Part print with two shaded views. Sizes in mm from the minimum x, y, z corner. A direction names the side the tool comes from. Round coordinates to 2 decimals unless told otherwise and drop trailing zeros. Loops run counter-clockwise (first coordinate to the right, second up) from the corner with the lowest first, then second, coordinate; pieces in that order, holes last. Notation, with made-up numbers: (87, 51.25) -> (107, 51.25) arc R23 ccw to (107, 63.25) -> close; hole circle Ø9 at (-19.75, 73). An arc over 180 degrees is marked (long way). Use a Markdown table: item, result. Add a question column.
Item 1: Cut at A-A, the plane z = 16.5. List the corners of the cut face in (x, y).
Item 2: Cut at B-B, the plane z = 69. List the corners of the cut face in (x, y), plus the area to 3 significant figures.
Item 3: Flat gauge pins, fed straight in: pin 1 (12 mm diameter, centred on y = 49.5, z = 14, fed in from +X); pin 2 (3 mm diameter, centred on x = 17.5, z = 39.5, fed in from +Y) (1 decimal); pin 3 (6 mm diameter, centred on x = 18.5, y = 35, fed in from +Z); pin 4 (8 mm diameter, centred on x = 31, y = 8, fed in from -Z). Where does each tip first touch, or does it go through?
Item 4: Probe line 1 (X direction, y = 15.5, z = 17) (1 decimal); line 2 (Z direction, x = 26, y = 18); line 3 (Y direction, x = 58, z = 15) (1 decimal). List the from-to ranges inside material, lowest first. Write a range as [from, to].
Item 5: Two-plate mould, pull along Y, no slides. Class the marked faces 3, 4, 5 and 6: pulls with the +Y half, pulls with the -Y half, needs draft (parallel to the pull), parting line crosses it, or undercut.
Item 6: Which spindle directions (+Z, -Z, +X, -X, +Y, -Y) get a long thin tool onto all of the face, cutting with end or side? Do the marked faces 1 and 2. Say none if no direction does.
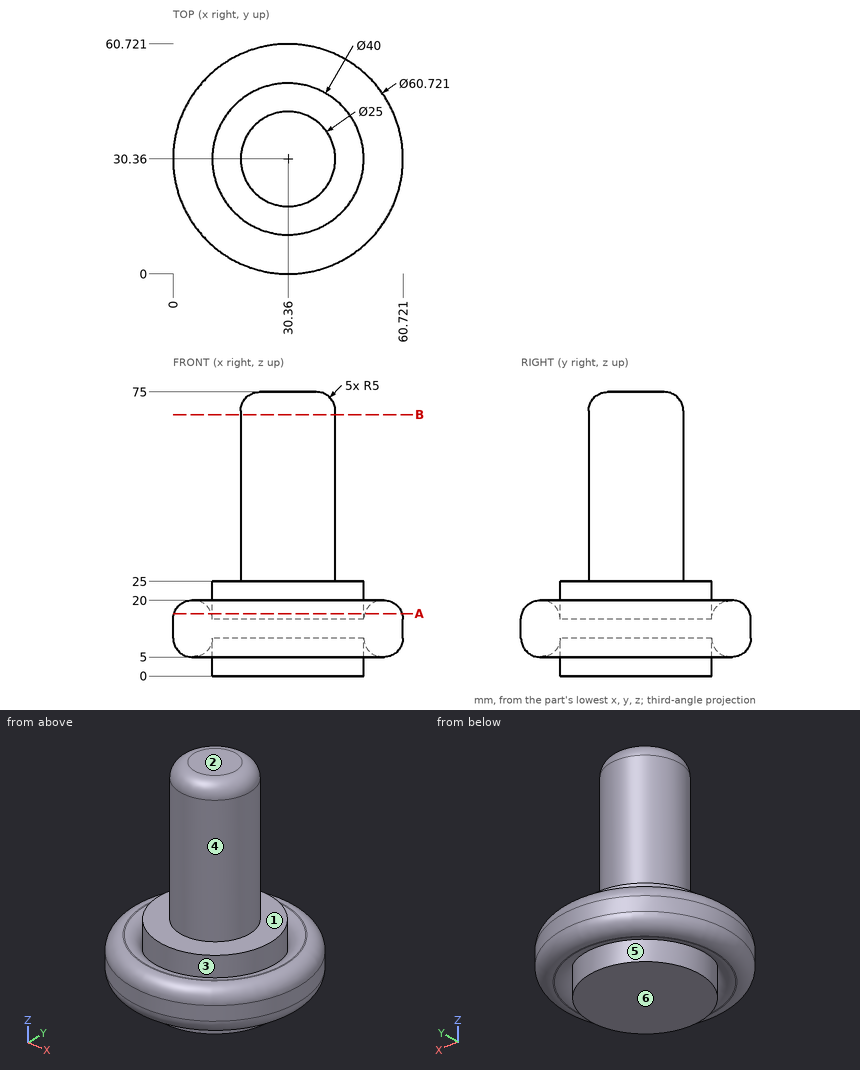
A:
| question | item | result |
|---|---|---|
| 1 | outline | circle Ø60.26 at (30.36, 30.36); circle Ø40 at (30.36, 30.36); hole circle Ø40.46 at (30.36, 30.36) |
| 2 | outline | circle Ø25 at (30.36, 30.36) |
| 2 | area | 491 mm^2 |
| 3 | pin 1 | stops at x = 57.73 |
| 3 | pin 2 | stops at y = 35.6 |
| 3 | pin 3 | stops at z = 74.47 |
| 3 | pin 4 | stops at z = 0 |
| 4 | line 1 | x = [4.4, 16.4], [17, 43.7], [44.4, 56.4] |
| 4 | line 2 | z = [0, 25] |
| 4 | line 3 | y = [17.8, 42.9] |
| 5 | face 3 | undercut |
| 5 | face 4 | parting line crosses it |
| 5 | face 5 | undercut |
| 5 | face 6 | needs draft |
| 6 | face 1 | +Z |
| 6 | face 2 | +Z, +X, -X, +Y, -Y |
